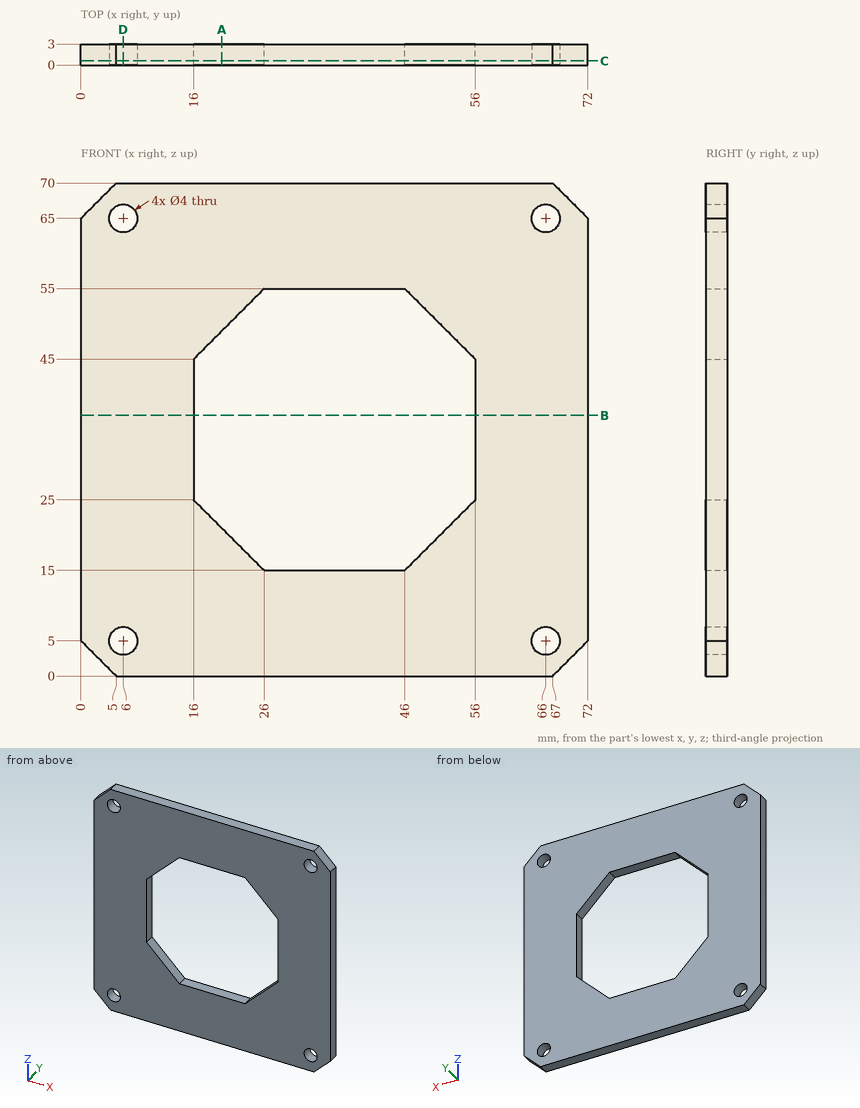
Part print with two shaded views. Sizes in mm from the minimum x, y, z corner. Coordinates: 2 decimals unless noted, no trailing zeros. Order: outer loops, then holes, each group sorted by start corner. A loop starts at its lowest first (then second) coordinate and runs counter-clockwise, first axis right, second up. Notation, with made-up numbers: M 57.25,48.25 L 100.25,48.25 A28 cw 100.25,80.25 Z; hole C -10.75,43.25 d7. An arc over 180 degrees is marked long. One line per question, with ' | ' between items. Start each with the question number.
1. Cut at A-A (x = 20). Write the cut outline in (y, z).
2. Cut at C-C (y = 0.6). Write the cut outline in (x, z).
3. Cut at B-B (z = 37). Write the cut outline in (x, y).
4. Wall check: line 1 along X through (y, z) = (2.35, 5); line 2 along Z through (x, y) = (66, 1.3); line 3 along Z through (x, y) = (17.5, 2.7). Give the ranges that are in metal, low to high. Write a range as [from, to].
5. Cut at D-D (x = 6). Write the cut outline in (y, z).
The answers:
1) outline: M 0,0 L 3,0 L 3,21 L 0,21 Z; M 0,49 L 3,49 L 3,70 L 0,70 Z
2) outline: M 0,5 L 5,0 L 67,0 L 72,5 L 72,65 L 67,70 L 5,70 L 0,65 Z; hole C 6,5 d4; hole C 6,65 d4; hole M 16,25 L 26,15 L 46,15 L 56,25 L 56,45 L 46,55 L 26,55 L 16,45 Z; hole C 66,5 d4; hole C 66,65 d4
3) outline: M 0,0 L 16,0 L 16,3 L 0,3 Z; M 56,0 L 72,0 L 72,3 L 56,3 Z
4) line 1: x = [0, 4], [8, 64], [68, 72] | line 2: z = [0, 3], [7, 63], [67, 70] | line 3: z = [0, 23.5], [46.5, 70]
5) outline: M 0,0 L 3,0 L 3,3 L 0,3 Z; M 0,7 L 3,7 L 3,63 L 0,63 Z; M 0,67 L 3,67 L 3,70 L 0,70 Z
